from build123d import *

# Parameters (mm, degrees)
SKETCH_1_R          = 27
SKETCH_1_R_2        = 10.5
SKETCH_1_R_3        = 2.6
EXTRUDE_1_DEPTH     = 3
SKETCH_3_R          = 2.6
CUT_EXTRUDE_2_DEPTH = 3


with BuildPart() as part:
    # 草图1 → 凸台-拉伸1 (new body)
    with BuildSketch(Plane.XY):
        Circle(SKETCH_1_R)
        Circle(SKETCH_1_R_2, mode=Mode.SUBTRACT)
        with Locations((0, 22.5)):
            Circle(SKETCH_1_R_3, mode=Mode.SUBTRACT)
        with Locations((19.485571585, 11.25)):
            Circle(SKETCH_1_R_3, mode=Mode.SUBTRACT)
        with Locations((19.485571585, -11.25)):
            Circle(SKETCH_1_R_3, mode=Mode.SUBTRACT)
        with Locations((0, -22.5)):
            Circle(SKETCH_1_R_3, mode=Mode.SUBTRACT)
        with Locations((-19.485571585, -11.25)):
            Circle(SKETCH_1_R_3, mode=Mode.SUBTRACT)
        with Locations((-19.485571585, 11.25)):
            Circle(SKETCH_1_R_3, mode=Mode.SUBTRACT)
    extrude(amount=EXTRUDE_1_DEPTH)

    # 草图3 → 切除-拉伸2 (cut)
    with BuildSketch(Plane.XY.offset(3)):
        with Locations((11.25, 19.485571585)):
            Circle(SKETCH_3_R)
        with Locations((22.5, 0)):
            Circle(SKETCH_3_R)
        with Locations((11.25, -19.485571585)):
            Circle(SKETCH_3_R)
        with Locations((-11.25, -19.485571585)):
            Circle(SKETCH_3_R)
        with Locations((-22.5, 0)):
            Circle(SKETCH_3_R)
        with Locations((-11.25, 19.485571585)):
            Circle(SKETCH_3_R)
    extrude(amount=-CUT_EXTRUDE_2_DEPTH, mode=Mode.SUBTRACT)


solid = part.part
The model under review builds one solid part; all positions refer to its coordinate system, in mm. Round coordinates to 2 decimals unless told otherwise and drop trailing zeros. Write each loop counter-clockwise with the first axis right and the second up, starting at its lowest first coordinate (ties: lowest second). Pieces come first, ordered by that corner, then holes. Notation, with made-up numbers: (-19, -12.75) - (8, -12.75) arc R14 ccw to (8, 6.25) - close; hole circle Ø7 at (62.5, 47.5). An arc over 180 degrees is marked (long way). One line per item, written item: value. Start each with the question number.
1. Consider section B-B on y = -7. Write out the cut boundary in (x, z), and give its area (3 significant figures).
2. Consider section C-C on x = -11.25. Write out the cut boundary in (y, z).
3. Clearance check with flat-ended pins moving along their axes: P1, Ø4.5, axis at x = -22.5, y = 0, coming from the -Z side; P2, Ø1, axis at y = 7, z = 2.5, coming from the +X side. State where each tip first meets the part, or that it passes through.
4. The part is to be moulded in two halves that separate along Y. For faces 1 (the face through (13.65, 18.49, 1.52)), 2 (the face through (12, 0, 0)), 3 (the face through (-5.85, -26.36, 1.48)), say which applies: released by +Y, released by -Y, zero draft, split by the parting line, or undercut.
5. Consider section A-A on x = -5. Write out the cut boundary in (y, z), and give its area (3 significant figures).
6. To check wall thickness, follow L1, parallel to Y at x = 0, z = 2.3; L2, parallel to Y at x = 18, z = 1.95; L3, parallel to Y at x = -9, z = 0.25. State the ranges of each line that lie inside material, in increasing order. Write a range as from..to.
7. Consider section D-D on y = -17.5. Write out the cut boundary in (x, z), and give its area (3 significant figures).
Checks:
1. outline: (-26.08, 0) - (-7.83, 0) - (-7.83, 3) - (-26.08, 3) - close; (7.83, 0) - (26.08, 0) - (26.08, 3) - (7.83, 3) - close
1. area: 110 mm^2
2. outline: (-24.54, 0) - (-22.09, 0) - (-22.09, 3) - (-24.54, 3) - close; (-16.89, 0) - (16.89, 0) - (16.89, 3) - (-16.89, 3) - close; (22.09, 0) - (24.54, 0) - (24.54, 3) - (22.09, 3) - close
3. P1: passes through
3. P2: stops at x = 26.21
4. face 1: undercut
4. face 2: zero draft
4. face 3: split by the parting line
5. outline: (-26.53, 0) - (-9.23, 0) - (-9.23, 3) - (-26.53, 3) - close; (9.23, 0) - (26.53, 0) - (26.53, 3) - (9.23, 3) - close
5. area: 104 mm^2
6. L1: y = -27..-25.1, -19.9..-10.5, 10.5..19.9, 25.1..27
6. L2: y = -20.12..-13.38, -9.12..9.12, 13.38..20.12
6. L3: y = -25.46..-20.79, -18.18..-5.41, 5.41..18.18, 20.79..25.46
7. outline: (-20.56, 0) - (-12.93, 0) - (-12.93, 3) - (-20.56, 3) - close; (-9.57, 0) - (9.57, 0) - (9.57, 3) - (-9.57, 3) - close; (12.93, 0) - (20.56, 0) - (20.56, 3) - (12.93, 3) - close
7. area: 103 mm^2
